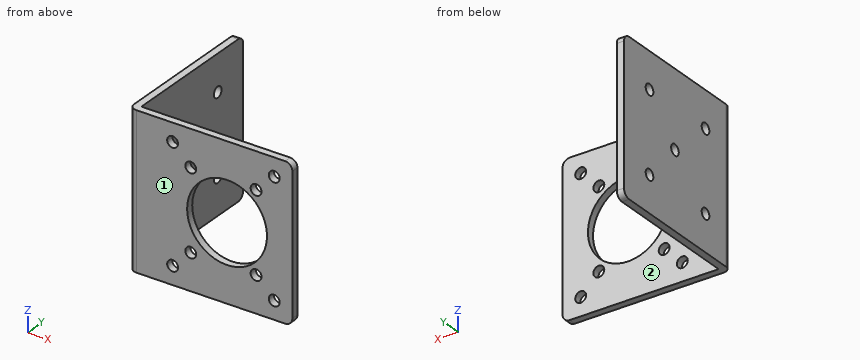
```python
from build123d import *

# Parameters (mm, degrees)
BOSS_EXTRUDE1_DEPTH = 42
FILLET1_R           = 2
FILLET2_R           = 2
CUT_EXTRUDE1_REACH  = 75.41
SKETCH3_R           = 11
SKETCH3_R_2         = 1.5
CUT_EXTRUDE2_REACH  = 75.328
SKETCH4_R           = 1.5


with BuildPart() as part:
    # Sketch1 → Boss-Extrude1 (new body)
    with BuildSketch(Plane.XY):
        Polygon((0, 0), (45, 0), (45, 2), (2, 2), (2, 42), (0, 42), align=None)
    extrude(amount=-BOSS_EXTRUDE1_DEPTH)

    # Fillet1
    fillet1_edges = [part.edges().sort_by_distance(p)[0] for p in [
        (0, 0, -21),
    ]]
    fillet(fillet1_edges, radius=FILLET1_R)

    # Fillet2
    fillet2_edges = [part.edges().sort_by_distance(p)[0] for p in [
        (45, 1, -42),
        (1, 42, -42),
        (1, 42, 0),
        (45, 1, 0),
    ]]
    fillet(fillet2_edges, radius=FILLET2_R)

    # Sketch3 → Cut-Extrude1 (cut, up to next)
    with BuildSketch(Plane(origin=(0, 2, 0), x_dir=(1, 0, 0), z_dir=(0, 1, 0)), mode=Mode.PRIVATE) as cut_extrude1_sk1:
        with Locations(Location((27, 21, 0), (0, 0, 180))):
            Circle(SKETCH3_R)
    cut_extrude1_tool1 = extrude(cut_extrude1_sk1.sketch, amount=-CUT_EXTRUDE1_REACH, mode=Mode.PRIVATE) & part.part
    # Sketch3 → Cut-Extrude1 (cut, up to next)
    with BuildSketch(Plane(origin=(0, 2, 0), x_dir=(1, 0, 0), z_dir=(0, 1, 0)), mode=Mode.PRIVATE) as cut_extrude1_sk2:
        with Locations(Location((40, 37, 0), (0, 0, 180))):
            Circle(SKETCH3_R_2)
    cut_extrude1_tool2 = extrude(cut_extrude1_sk2.sketch, amount=-CUT_EXTRUDE1_REACH, mode=Mode.PRIVATE) & part.part
    # Sketch3 → Cut-Extrude1 (cut, up to next)
    with BuildSketch(Plane(origin=(0, 2, 0), x_dir=(1, 0, 0), z_dir=(0, 1, 0)), mode=Mode.PRIVATE) as cut_extrude1_sk3:
        with Locations(Location((40, 5, 0), (0, 0, 180))):
            Circle(SKETCH3_R_2)
    cut_extrude1_tool3 = extrude(cut_extrude1_sk3.sketch, amount=-CUT_EXTRUDE1_REACH, mode=Mode.PRIVATE) & part.part
    # Sketch3 → Cut-Extrude1 (cut, up to next)
    with BuildSketch(Plane(origin=(0, 2, 0), x_dir=(1, 0, 0), z_dir=(0, 1, 0)), mode=Mode.PRIVATE) as cut_extrude1_sk4:
        with Locations(Location((35, 32, 0), (0, 0, 180))):
            Circle(SKETCH3_R_2)
    cut_extrude1_tool4 = extrude(cut_extrude1_sk4.sketch, amount=-CUT_EXTRUDE1_REACH, mode=Mode.PRIVATE) & part.part
    # Sketch3 → Cut-Extrude1 (cut, up to next)
    with BuildSketch(Plane(origin=(0, 2, 0), x_dir=(1, 0, 0), z_dir=(0, 1, 0)), mode=Mode.PRIVATE) as cut_extrude1_sk5:
        with Locations(Location((35, 10, 0), (0, 0, 180))):
            Circle(SKETCH3_R_2)
    cut_extrude1_tool5 = extrude(cut_extrude1_sk5.sketch, amount=-CUT_EXTRUDE1_REACH, mode=Mode.PRIVATE) & part.part
    # Sketch3 → Cut-Extrude1 (cut, up to next)
    with BuildSketch(Plane(origin=(0, 2, 0), x_dir=(1, 0, 0), z_dir=(0, 1, 0)), mode=Mode.PRIVATE) as cut_extrude1_sk6:
        with Locations(Location((17, 10, 0), (0, 0, 180))):
            Circle(SKETCH3_R_2)
    cut_extrude1_tool6 = extrude(cut_extrude1_sk6.sketch, amount=-CUT_EXTRUDE1_REACH, mode=Mode.PRIVATE) & part.part
    # Sketch3 → Cut-Extrude1 (cut, up to next)
    with BuildSketch(Plane(origin=(0, 2, 0), x_dir=(1, 0, 0), z_dir=(0, 1, 0)), mode=Mode.PRIVATE) as cut_extrude1_sk7:
        with Locations(Location((17, 32, 0), (0, 0, 180))):
            Circle(SKETCH3_R_2)
    cut_extrude1_tool7 = extrude(cut_extrude1_sk7.sketch, amount=-CUT_EXTRUDE1_REACH, mode=Mode.PRIVATE) & part.part
    # Sketch3 → Cut-Extrude1 (cut, up to next)
    with BuildSketch(Plane(origin=(0, 2, 0), x_dir=(1, 0, 0), z_dir=(0, 1, 0)), mode=Mode.PRIVATE) as cut_extrude1_sk8:
        with Locations(Location((12, 37, 0), (0, 0, 180))):
            Circle(SKETCH3_R_2)
    cut_extrude1_tool8 = extrude(cut_extrude1_sk8.sketch, amount=-CUT_EXTRUDE1_REACH, mode=Mode.PRIVATE) & part.part
    # Sketch3 → Cut-Extrude1 (cut, up to next)
    with BuildSketch(Plane(origin=(0, 2, 0), x_dir=(1, 0, 0), z_dir=(0, 1, 0)), mode=Mode.PRIVATE) as cut_extrude1_sk9:
        with Locations(Location((12, 5, 0), (0, 0, 180))):
            Circle(SKETCH3_R_2)
    cut_extrude1_tool9 = extrude(cut_extrude1_sk9.sketch, amount=-CUT_EXTRUDE1_REACH, mode=Mode.PRIVATE) & part.part
    add(cut_extrude1_tool1.solids().sort_by_distance((27, 2, -21))[0], mode=Mode.SUBTRACT)
    add(cut_extrude1_tool2.solids().sort_by_distance((40, 2, -37))[0], mode=Mode.SUBTRACT)
    add(cut_extrude1_tool3.solids().sort_by_distance((40, 2, -5))[0], mode=Mode.SUBTRACT)
    add(cut_extrude1_tool4.solids().sort_by_distance((35, 2, -32))[0], mode=Mode.SUBTRACT)
    add(cut_extrude1_tool5.solids().sort_by_distance((35, 2, -10))[0], mode=Mode.SUBTRACT)
    add(cut_extrude1_tool6.solids().sort_by_distance((17, 2, -10))[0], mode=Mode.SUBTRACT)
    add(cut_extrude1_tool7.solids().sort_by_distance((17, 2, -32))[0], mode=Mode.SUBTRACT)
    add(cut_extrude1_tool8.solids().sort_by_distance((12, 2, -37))[0], mode=Mode.SUBTRACT)
    add(cut_extrude1_tool9.solids().sort_by_distance((12, 2, -5))[0], mode=Mode.SUBTRACT)

    # Sketch4 → Cut-Extrude2 (cut, up to next)
    with BuildSketch(Plane(origin=(2, 0, 0), x_dir=(0, 0, -1), z_dir=(1, 0, 0)), mode=Mode.PRIVATE) as cut_extrude2_sk1:
        with Locations(Location((21, 22, 0), (0, 0, 90))):
            Circle(SKETCH4_R)
    cut_extrude2_tool1 = extrude(cut_extrude2_sk1.sketch, amount=-CUT_EXTRUDE2_REACH, mode=Mode.PRIVATE) & part.part
    # Sketch4 → Cut-Extrude2 (cut, up to next)
    with BuildSketch(Plane(origin=(2, 0, 0), x_dir=(0, 0, -1), z_dir=(1, 0, 0)), mode=Mode.PRIVATE) as cut_extrude2_sk2:
        with Locations(Location((10, 32, 0), (0, 0, 90))):
            Circle(SKETCH4_R)
    cut_extrude2_tool2 = extrude(cut_extrude2_sk2.sketch, amount=-CUT_EXTRUDE2_REACH, mode=Mode.PRIVATE) & part.part
    # Sketch4 → Cut-Extrude2 (cut, up to next)
    with BuildSketch(Plane(origin=(2, 0, 0), x_dir=(0, 0, -1), z_dir=(1, 0, 0)), mode=Mode.PRIVATE) as cut_extrude2_sk3:
        with Locations(Location((32, 32, 0), (0, 0, 90))):
            Circle(SKETCH4_R)
    cut_extrude2_tool3 = extrude(cut_extrude2_sk3.sketch, amount=-CUT_EXTRUDE2_REACH, mode=Mode.PRIVATE) & part.part
    # Sketch4 → Cut-Extrude2 (cut, up to next)
    with BuildSketch(Plane(origin=(2, 0, 0), x_dir=(0, 0, -1), z_dir=(1, 0, 0)), mode=Mode.PRIVATE) as cut_extrude2_sk4:
        with Locations(Location((10, 10, 0), (0, 0, 90))):
            Circle(SKETCH4_R)
    cut_extrude2_tool4 = extrude(cut_extrude2_sk4.sketch, amount=-CUT_EXTRUDE2_REACH, mode=Mode.PRIVATE) & part.part
    # Sketch4 → Cut-Extrude2 (cut, up to next)
    with BuildSketch(Plane(origin=(2, 0, 0), x_dir=(0, 0, -1), z_dir=(1, 0, 0)), mode=Mode.PRIVATE) as cut_extrude2_sk5:
        with Locations(Location((32, 10, 0), (0, 0, 90))):
            Circle(SKETCH4_R)
    cut_extrude2_tool5 = extrude(cut_extrude2_sk5.sketch, amount=-CUT_EXTRUDE2_REACH, mode=Mode.PRIVATE) & part.part
    add(cut_extrude2_tool1.solids().sort_by_distance((2, 22, -21))[0], mode=Mode.SUBTRACT)
    add(cut_extrude2_tool2.solids().sort_by_distance((2, 32, -10))[0], mode=Mode.SUBTRACT)
    add(cut_extrude2_tool3.solids().sort_by_distance((2, 32, -32))[0], mode=Mode.SUBTRACT)
    add(cut_extrude2_tool4.solids().sort_by_distance((2, 10, -10))[0], mode=Mode.SUBTRACT)
    add(cut_extrude2_tool5.solids().sort_by_distance((2, 10, -32))[0], mode=Mode.SUBTRACT)


solid = part.part
```
For this review, take the finished solid that the model builds, in its own axes (mm). Face numbers are marked on the shaded views. A direction names the side the tool comes from. Coordinates: 2 decimals unless noted, no trailing zeros. Loops run counter-clockwise (first coordinate to the right, second up) from the corner with the lowest first, then second, coordinate; pieces in that order, holes last.
1. Add section A-A, the plane z = -21. Give the boundary of the cut face in (x, y), then the cut area to 3 significant figures.
2. For line 1 (Z direction, x = 12, y = 0.6); line 2 (Y direction, x = 2.5, z = -28), list the stretches that pass through material, from the lowest coordinate up.
3. For the marked faces 1 and 2, list the 3-axis set-ups (+Z, -Z, +X, -X, +Y, -Y) from which the entire face can be reached by the end or side of a thin tool; tool diameter is ignored.
4. Add section B-B, the plane y = 22. Give the boundary of the cut face in (x, z), then the cut area to 3 significant figures.
5. Add section D-D, the plane y = 10. Give the boundary of the cut face in (x, z).
6. Add section C-C, the plane x = 12. Give the boundary of the cut face in (y, z), then the cut area to 3 significant figures.
7. Insertion check: P1, Ø12, axis at y = 14, z = -26, coming from the +X side; P2, Ø4, axis at y = 22, z = -21, coming from the -X side; P3, Ø12.5, axis at x = 21.5, z = -16, coming from the +Y side; P4, Ø2.5, axis at x = 35, z = -10, coming from the +Y side. Each pin has a flat end and moves straight along its axis. Give the tip position at first contact, or say it passes through.
Result:
1. outline: (0, 2) arc R2 ccw to (2, 0) - (16, 0) - (16, 2) - (2, 2) - (2, 20.5) - (0, 20.5) - close; (0, 23.5) - (2, 23.5) - (2, 42) - (0, 42) - close; (38, 0) - (45, 0) - (45, 2) - (38, 2) - close
1. area: 119 mm2
2. line 1: z = -42 to -38.5, -35.5 to -6.5, -3.5 to 0
2. line 2: y = 0 to 2
3. face 1: +Z, -Z, +X, -X, -Y
3. face 2: +Z, -Z, +X, +Y
4. outline: (0, -42) - (2, -42) - (2, -22.5) - (0, -22.5) - close; (0, -19.5) - (2, -19.5) - (2, 0) - (0, 0) - close
4. area: 78.0 mm2
5. outline: (0, -42) - (2, -42) - (2, -33.5) - (0, -33.5) - close; (0, -30.5) - (2, -30.5) - (2, -11.5) - (0, -11.5) - close; (0, -8.5) - (2, -8.5) - (2, 0) - (0, 0) - close
6. outline: (0, -42) - (2, -42) - (2, -38.5) - (0, -38.5) - close; (0, -35.5) - (2, -35.5) - (2, -6.5) - (0, -6.5) - close; (0, -3.5) - (2, -3.5) - (2, 0) - (0, 0) - close
6. area: 72.0 mm2
7. P1: stops at x = 2
7. P2: stops at x = 0
7. P3: stops at y = 2
7. P4: passes through
